Geometry: see drawing. Coordinates: mm, zero at the bounding-box minimum. A direction names the side the tool comes from. Give positions to 0.01 mm unless a question says otherwise; leave off trailing zeros. Write each loop counter-clockwise with the first axis right and the second up, starting at its lowest first coordinate (ties: lowest second). Pieces come first, ordered by that corner, then holes. Notation, with made-up numbers: (-19.5, 13) - (17.5, 13) arc R17 cw to (17.5, 30) - close; hole circle Ø8 at (10.25, 84.25). An arc over 180 degrees is marked (long way). Return JSON: item names as keys, results as strings.
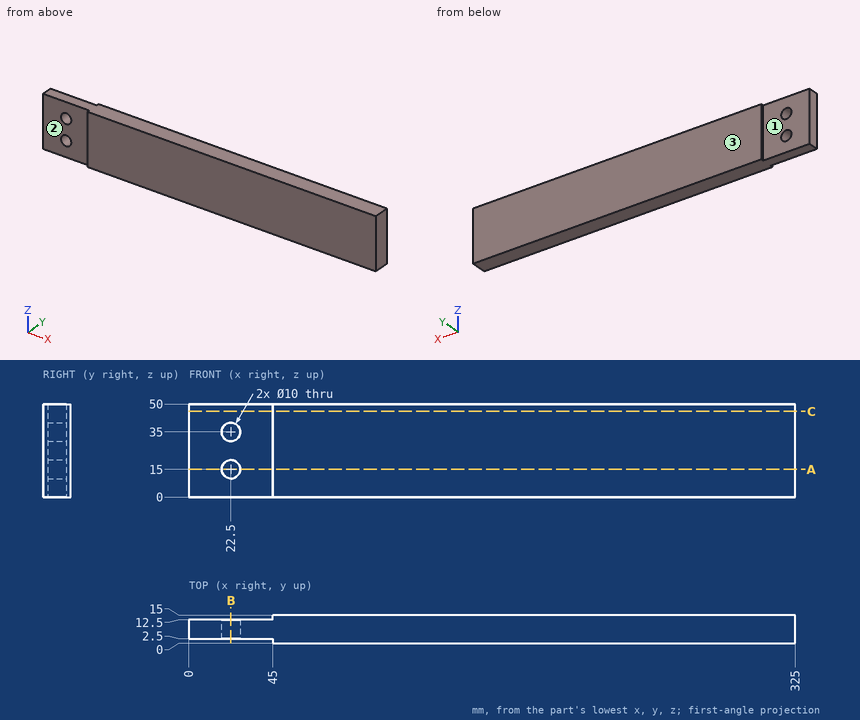
Q1. Section query B-B, the plane x = 22.5. Return the cut outline in (y, z), plus the area to 3 significant figures.
Answer key:
{"outline": "(2.5, 0) - (12.5, 0) - (12.5, 10) - (2.5, 10) - close; (2.5, 20) - (12.5, 20) - (12.5, 30) - (2.5, 30) - close; (2.5, 40) - (12.5, 40) - (12.5, 50) - (2.5, 50) - close", "area": "300 mm^2"}
Q2. Section query C-C, the plane z = 46. Return the cut outline in (x, y), plus the area to 3 significant figures.
Answer key:
{"outline": "(0, 2.5) - (45, 2.5) - (45, 0) - (325, 0) - (325, 15) - (45, 15) - (45, 12.5) - (0, 12.5) - close", "area": "4,650 mm^2"}
Q3. Section query A-A, the plane z = 15. Return the cut outline in (x, y).
Answer key:
{"outline": "(0, 2.5) - (17.5, 2.5) - (17.5, 12.5) - (0, 12.5) - close; (27.5, 2.5) - (45, 2.5) - (45, 0) - (325, 0) - (325, 15) - (45, 15) - (45, 12.5) - (27.5, 12.5) - close"}
Q4. Material intervals for probe 1 along Z at (x, y) = (22.5, 9); probe 2 along X at (y, z) = (6.5, 35); probe 3 along X at (y, z) = (1.75, 22), sorted ascending. Write a range as [from, to].
Answer key:
{"probe 1": "z = [0, 10], [20, 30], [40, 50]", "probe 2": "x = [0, 17.5], [27.5, 325]", "probe 3": "x = [45, 325]"}
Q5. Set-up query: the marked faces 1, 2 and 3. Return all of +Z, -Z, +X, -X, +Y, -Y with unobstructed straight access to the full face (end or side cutting, diameter ignored); none if empty.
Answer key:
{"face 1": "+Z, -Z, -X, +Y", "face 2": "+Z, -Z, -X, -Y", "face 3": "+Z, -Z, +X, -X, +Y"}
Q6. Pin query (flat end, axial travel): P1, Ø1, axis at y = 8, z = 29.5, coming from the -X side; P2, Ø16, axis at x = 22.5, z = 35, coming from the +Y side; P3, Ø1.2, axis at y = 13.5, z = 32.5, coming from the -X side. Return the tip coordinate at first contact, or that it passes through.
Answer key:
{"P1": "stops at x = 0", "P2": "stops at y = 12.5", "P3": "stops at x = 45"}
